Input: part model. Units: mm. Frame: model coordinates. Coordinates: 2 decimals unless noted, no trailing zeros. Loops run counter-clockwise (first coordinate to the right, second up) from the corner with the lowest first, then second, coordinate; pieces in that order, holes last. Notation, with made-up numbers: (40.5, 78.25) - (90.5, 78.25) arc R15 cw to (90.5, 104.25) - close; hole circle Ø3 at (-3.75, -7). An arc over 180 degrees is marked (long way). Use a Markdown table: item, result. Add a question column.
1. Section query C-C on z = 1.5. Return the cut outline in (x, y).
2. Ray query, L1, parallel to X at y = 0.25, z = 49.5; L2, parallel to Z at x = 29, y = 0.7 (3 decimals); L3, parallel to X at y = -0.45, z = -55. Return the intervals inside material, ascending. Write a range as [from, to].
3. Section query A-A on y = 0.45. State how many separate pieces and enclosed holes the cut face has, then the cut area to 3 significant figures.
4. Contact query for flat-ended pins moving along their axis: P1, Ø6.5, axis at x = 149.53, z = 82.68, coming from the -Y side; P2, Ø1, axis at y = 0.5, z = 12, coming from the +X side; P3, Ø1.6, axis at x = -1.5, y = -0.5, coming from the -Z side (3 decimals). Output: stop coordinate, or through.
5. Section query B-B on x = -291. Return the cut outline in (y, z) (1 decimal), then the cut area to 3 significant figures.
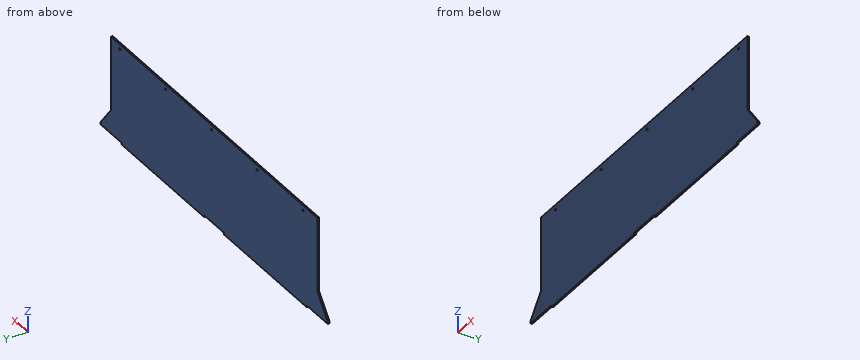
```python
from build123d import *

# Parameters (mm, degrees)
SKETCH1_W           = 635.3556
SKETCH1_H           = 184.15
BOSS_EXTRUDE1_DEPTH = 1.5875
SKETCH2_W           = 254
SKETCH2_H           = 3.175
BOSS_EXTRUDE2_DEPTH = 3.175
BOSS_EXTRUDE3_DEPTH = 3.175
CUT_EXTRUDE1_DEPTH  = 10
LPATTERN1_COUNT     = 5
LPATTERN1_PITCH     = 140.97


with BuildPart() as part:
    # Sketch1 → Boss-Extrude1 (new, symmetric)
    with BuildSketch(Plane(origin=(0, 0, 0), x_dir=(1, 0, 0), z_dir=(0, 1, 0))):
        Rectangle(SKETCH1_W, SKETCH1_H)
    extrude(amount=BOSS_EXTRUDE1_DEPTH, both=True)

    # Sketch2 → Boss-Extrude2 (add)
    with BuildSketch(Plane(origin=(0, 0, -92.075), x_dir=(-1, 0, 0), z_dir=(0, 0, -1))):
        with Locations((-157.8229, 0)):
            Rectangle(SKETCH2_W, SKETCH2_H)
        with Locations((157.8229, 0)):
            Rectangle(SKETCH2_W, SKETCH2_H)
    extrude(amount=BOSS_EXTRUDE2_DEPTH)

    # Sketch3 → Boss-Extrude3 (add)
    with BuildSketch(Plane.XZ.offset(1.5875)):
        Polygon((317.6778, -92.075), (349.4278, -92.075), (349.4278, -87.3125), (317.6778, -47.625), align=None)
    boss_extrude3 = extrude(amount=-BOSS_EXTRUDE3_DEPTH)

    # Mirror1: Boss-Extrude3 across plane
    add(boss_extrude3.mirror(Plane(origin=(0, 0, 0), x_dir=(0, 0, 1), z_dir=(1, 0, 0))))

    # Sketch4 → Cut-Extrude1 (cut)
    with BuildSketch(Plane(origin=(0, 1.5875, 0), x_dir=(1, 0, 0), z_dir=(0, 1, 0))):
        with BuildLine():
            ThreePointArc((292.5248, -82.677), (289.067908768, -81.245108768), (290.4998, -84.702))
            Line((290.4998, -84.702), (290.4998, -82.677))
            Line((290.4998, -82.677), (292.5248, -82.677))
        make_face()
        with BuildLine():
            Line((290.4998, -82.677), (290.4998, -84.702))
            ThreePointArc((290.4998, -84.702), (291.931691232, -84.108891232), (292.5248, -82.677))
            Line((292.5248, -82.677), (290.4998, -82.677))
        make_face()
    cut_extrude1 = extrude(amount=-CUT_EXTRUDE1_DEPTH, mode=Mode.SUBTRACT)

    # LPattern1: Cut-Extrude1 ×5
    with Locations(*[(-i * LPATTERN1_PITCH, 0, 0) for i in range(1, LPATTERN1_COUNT)]):
        add(cut_extrude1, mode=Mode.SUBTRACT)


solid = part.part
```
Resolved:
| question | item | result |
|---|---|---|
| 1 | outline | (-317.68, -1.59) - (317.68, -1.59) - (317.68, 1.59) - (-317.68, 1.59) - close |
| 2 | L1 | [-317.68, 317.68] |
| 2 | L2 | [-92.075, 92.075] |
| 2 | L3 | [-323.58, 323.58] |
| 3 | separate pieces | 1 |
| 3 | enclosed holes | 5 |
| 3 | area | 120,000 mm² |
| 4 | P1 | y = -1.59 |
| 4 | P2 | x = 317.68 |
| 4 | P3 | z = -92.075 |
| 5 | outline | (-1.6, -92.1) - (1.6, -92.1) - (1.6, 92.1) - (-1.6, 92.1) - close |
| 5 | area | 585 mm² |
